Job drawing, mm, ordinate dimensions from the low corner. One solid piece. A direction names the side the tool comes from. Give positions to 0.01 mm unless a question says otherwise; leave off trailing zeros. Order: outer loops, then holes, each group sorted by start corner. A loop starts at its lowest first (then second) coordinate and runs counter-clockwise, first axis right, second up. Notation, with made-up numbers: (36.25, 34.5) -> (79.25, 34.5) arc R25 cw to (79.25, 61.5) -> close; hole circle Ø7 at (6.25, 89). An arc over 180 degrees is marked (long way). Write item = value, one per line. Start each with the question number.
(1) Flat gauge pins, fed straight in: pin 1 (0.8 mm diameter, centred on x = 12, y = 0.5, fed in from +Z); pin 2 (2.5 mm diameter, centred on x = 11.5, y = 10, fed in from +Z); pin 3 (3.5 mm diameter, centred on x = 12, y = 25, fed in from +Z); pin 4 (1.5 mm diameter, centred on y = 32, z = 3.5, fed in from +X). Where does each tip first touch, or does it go through?
(2) Probe line 1 along X through (y, z) = (20, 0.9); line 2 along Z through (x, y) = (13.75, 27). List the from-to ranges inside material, lowest first. Write a range as from..to.
(3) Which spindle directions (+Z, -Z, +X, -X, +Y, -Y) get a long thin tool onto all of the face, cutting with end or side? Do the marked faces 1, 2 and 3. Say none if no direction does.
(4) Saw through at A-A, the plane z = 10. List the corners of the cut face in (x, y), then the cut area to 3 significant figures.
(5) Saw through at D-D, the plane x = 3.75. List the corners of the cut face in (y, z), then the cut area to 3 significant figures.
(6) Saw through at B-B, the plane y = 10. List the corners of the cut face in (x, z), then the cut area to 4 significant figures.
(7) Saw through at C-C, the plane y = 25. List the corners of the cut face in (x, z), then the cut area to 4 significant figures.
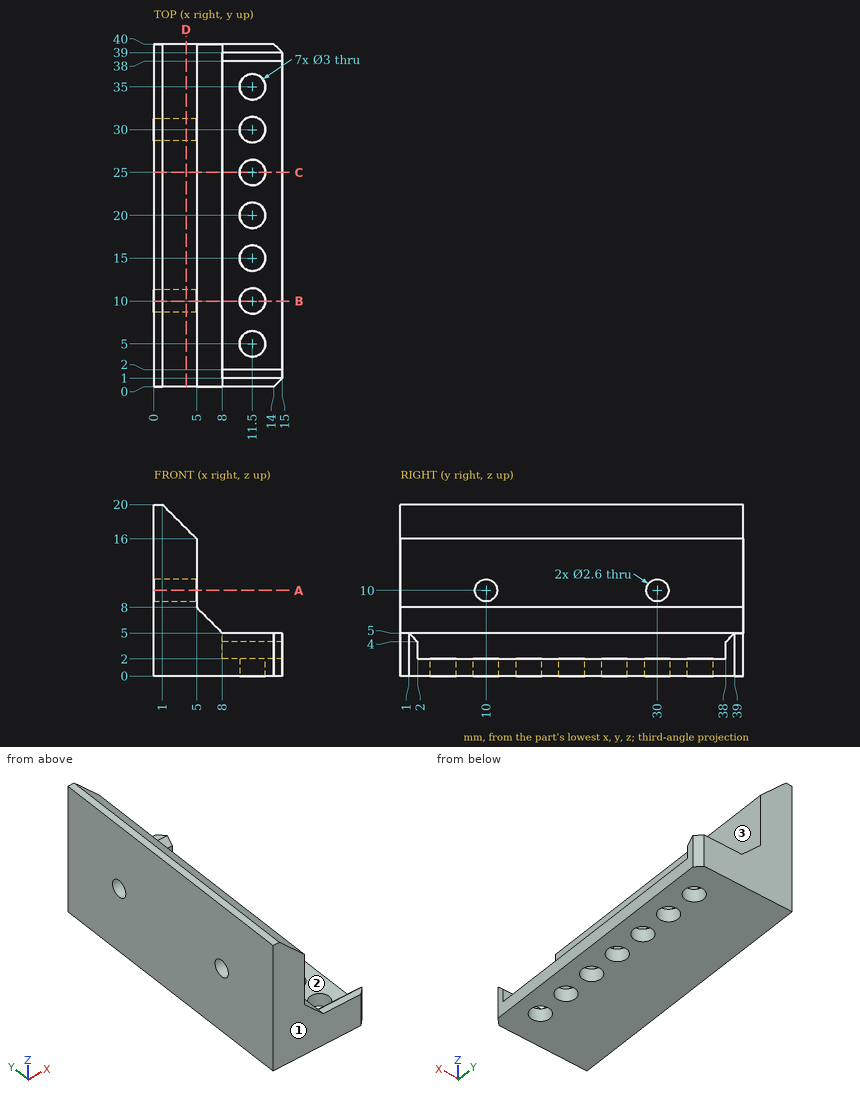
Results list:
q1.pin_1 = 5
q1.pin_2 = through
q1.pin_3 = 2
q1.pin_4 = 8
q2.line_1 = 0..10, 13..15
q2.line_2 = 0..2
q3.face_1 = +Z, -Z, +X, -X, -Y
q3.face_2 = +Z, +X
q3.face_3 = +Z, +X, +Y, -Y
q4.outline = (0, 0) -> (5, 0) -> (5, 8.7) -> (0, 8.7) -> close; (0, 11.3) -> (5, 11.3) -> (5, 28.7) -> (0, 28.7) -> close; (0, 31.3) -> (5, 31.3) -> (5, 40) -> (0, 40) -> close
q4.area = 174 mm^2
q5.outline = (0, 0) -> (40, 0) -> (40, 17.25) -> (0, 17.25) -> close; hole circle Ø2.6 at (10, 10); hole circle Ø2.6 at (30, 10)
q5.area = 679 mm^2
q6.outline = (0, 0) -> (10, 0) -> (10, 2) -> (8, 2) -> (8, 5) -> (5, 8) -> (5, 8.7) -> (0, 8.7) -> close; (0, 11.3) -> (5, 11.3) -> (5, 16) -> (1, 20) -> (0, 20) -> close; (13, 0) -> (15, 0) -> (15, 2) -> (13, 2) -> close
q6.area = 106.5 mm^2
q7.outline = (0, 0) -> (10, 0) -> (10, 2) -> (8, 2) -> (8, 5) -> (5, 8) -> (5, 16) -> (1, 20) -> (0, 20) -> close; (13, 0) -> (15, 0) -> (15, 2) -> (13, 2) -> close
q7.area = 119.5 mm^2
